```python
from build123d import *

# Parameters (mm, degrees)
SKETCH_1_W          = 37
SKETCH_1_H          = 87
SKETCH_1_R          = 1.6
EXTRUDE_1_DEPTH     = 4
SKETCH_2_W          = 16.67
SKETCH_2_H          = 8
CUT_EXTRUDE_1_DEPTH = 48.439435073


with BuildPart() as part:
    # 草图1 → 凸台-拉伸1 (new body)
    with BuildSketch(Plane.XY):
        Rectangle(SKETCH_1_W, SKETCH_1_H)
        with Locations((-14, 33.5)):
            Circle(SKETCH_1_R, mode=Mode.SUBTRACT)
        with Locations((14, 33.5)):
            Circle(SKETCH_1_R, mode=Mode.SUBTRACT)
        with Locations((-14, -33.5)):
            Circle(SKETCH_1_R, mode=Mode.SUBTRACT)
        with Locations((14, -33.5)):
            Circle(SKETCH_1_R, mode=Mode.SUBTRACT)
    extrude(amount=EXTRUDE_1_DEPTH)

    # 草图2 → 切除-拉伸1 (cut, through all)
    with BuildSketch(Plane.XY.offset(4)):
        with Locations((-10.165, 15)):
            Rectangle(SKETCH_2_W, SKETCH_2_H)
        with Locations((10.165, -15)):
            Rectangle(SKETCH_2_W, SKETCH_2_H)
    extrude(amount=-CUT_EXTRUDE_1_DEPTH, mode=Mode.SUBTRACT)


solid = part.part
```
The model under review builds one solid part; all positions refer to its coordinate system, in mm. A direction names the side the tool comes from. Give positions to 0.01 mm unless a question says otherwise; leave off trailing zeros. Write each loop counter-clockwise with the first axis right and the second up, starting at its lowest first coordinate (ties: lowest second). Pieces come first, ordered by that corner, then holes.
(1) The part is to be moulded in two halves that separate along Y. For faces 1 (the flat face through (18.5, -31, 2)), 2 (the flat face through (0, 43.5, 2)), 3 (the flat face through (10, -19, 2)), 4 (the flat face through (-1.83, 15, 2)), say which applies: released by +Y, released by -Y, zero draft, split by the parting line, or undercut.
(2) For P1, Ø2.5, axis at x = -14, y = 33.5, coming from the +Z side, flat-tipped, find the tip position at first contact; note if it passes through.
(3) Consider section D-D, the plane z = 3.3. Give the boundary of the cut face in (x, y), and give its area (3 significant figures).
(4) Consider section A-A, the plane x = 14. Give the boundary of the cut face in (y, z).
(5) Consider section C-C, the plane x = -4.5. Give the boundary of the cut face in (y, z).
(6) Tool access review of faces 5 (the flat face through (-10, 19, 2)), 6 (the flat face through (0, -43.5, 2)), 7 (the flat face through (1.83, -15, 2)): name each direction out of +Z, -Z, +X, -X, +Y, -Y from which nothing blocks a thin tool from reaching the whole face with its end or side.
(7) Consider section B-B, the plane y = 33.5. Give the boundary of the cut face in (x, z), and give its area (3 significant figures).
(8) To check wall thickness, follow L1, parallel to Y at x = 14, z = 2.6; L2, parallel to Y at x = -14, z = 1.4; L3, parallel to Y at x = 2, z = 0.35. State the ranges of each line that lie inside material, in increasing order.
Returned:
1. face 1: zero draft
1. face 2: released by +Y
1. face 3: undercut
1. face 4: undercut
2. P1: passes through
3. outline: (-18.5, -43.5) - (18.5, -43.5) - (18.5, -19) - (1.83, -19) - (1.83, -11) - (18.5, -11) - (18.5, 43.5) - (-18.5, 43.5) - (-18.5, 19) - (-1.83, 19) - (-1.83, 11) - (-18.5, 11) - close; hole circle Ø3.2 at (-14, -33.5); hole circle Ø3.2 at (-14, 33.5); hole circle Ø3.2 at (14, -33.5); hole circle Ø3.2 at (14, 33.5)
3. area: 2,920 mm2
4. outline: (-43.5, 0) - (-35.1, 0) - (-35.1, 4) - (-43.5, 4) - close; (-31.9, 0) - (-19, 0) - (-19, 4) - (-31.9, 4) - close; (-11, 0) - (31.9, 0) - (31.9, 4) - (-11, 4) - close; (35.1, 0) - (43.5, 0) - (43.5, 4) - (35.1, 4) - close
5. outline: (-43.5, 0) - (11, 0) - (11, 4) - (-43.5, 4) - close; (19, 0) - (43.5, 0) - (43.5, 4) - (19, 4) - close
6. face 5: +Z, -Z, -X
6. face 6: +Z, -Z, +X, -X, -Y
6. face 7: +Z, -Z, +X
7. outline: (-18.5, 0) - (-15.6, 0) - (-15.6, 4) - (-18.5, 4) - close; (-12.4, 0) - (12.4, 0) - (12.4, 4) - (-12.4, 4) - close; (15.6, 0) - (18.5, 0) - (18.5, 4) - (15.6, 4) - close
7. area: 122 mm2
8. L1: y = -43.5 to -35.1, -31.9 to -19, -11 to 31.9, 35.1 to 43.5
8. L2: y = -43.5 to -35.1, -31.9 to 11, 19 to 31.9, 35.1 to 43.5
8. L3: y = -43.5 to -19, -11 to 43.5
